Geometry: final body of the model. Coordinates: model frame, mm. Face numbers are marked on the shaded views. A direction names the side the tool comes from. Give positions to 0.01 mm unless a question says otherwise; leave off trailing zeros. Write each loop counter-clockwise with the first axis right and the second up, starting at its lowest first coordinate (ties: lowest second). Pieces come first, ordered by that corner, then holes. Notation, with made-up numbers: (22.5, 23.25) -> (29.5, 23.25) arc R18 ccw to (29.5, 35.25) -> close; hole circle Ø3 at (48, 72.25). An arc over 180 degrees is marked (long way). Answer as a JSON object with one key per item and string values.
from build123d import *

# Parameters (mm, degrees)
F1_DEPTH        = 10
F0_R            = 2.9
F2_DEPTH        = 3
F3_R            = 6.5
F4_DEPTH        = 4
F5_R            = 5
F6_DEPTH        = 12
F7_DEPTH        = 2
F8_D            = 3.3
F8_DEPTH        = 13.8
F8_START        = 2
F8_TIP          = 0.9914200214
F9_DEPTH        = 1.4
F10_D           = 3.3
F10_DEPTH       = 8
F10_TIP         = 0.9914200214
F12_D           = 3.3
F12_DEPTH       = 8
F12_CSINK_D     = 6.72
F12_CSINK_ANGLE = 90
F12_TIP         = 0.9914200214


with BuildPart() as f1:
    # F0 (on Front) → F1 (new body)
    with BuildSketch(Plane.XZ):
        with BuildLine():
            Line((20.9, 37.9), (17.9, 37.9))
            Line((17.9, 37.9), (-17.9, 37.9))
            Line((-17.9, 37.9), (-20.9, 37.9))
            ThreePointArc((-20.9, 37.9), (-22.3142135624, 37.3142135624), (-22.9, 35.9))
            Line((-22.9, 35.9), (-22.9, 32.9))
            Line((-22.9, 32.9), (-22.9, -35.9))
            ThreePointArc((-22.9, -35.9), (-22.3142135624, -37.3142135624), (-20.9, -37.9))
            Line((-20.9, -37.9), (20.9, -37.9))
            ThreePointArc((20.9, -37.9), (22.3142135624, -37.3142135624), (22.9, -35.9))
            Line((22.9, -35.9), (22.9, 32.9))
            Line((22.9, 32.9), (22.9, 35.9))
            ThreePointArc((22.9, 35.9), (22.3142135624, 37.3142135624), (20.9, 37.9))
        make_face()
        Polygon((7.4256842194, -31), (10.7743157806, -31), (12.4486315613, -33.9), (10.7743157806, -36.8), (7.4256842194, -36.8), (5.7513684387, -33.9), align=None, mode=Mode.SUBTRACT)
        Polygon((-16.2256842194, 36.8), (-14.5513684387, 33.9), (-16.2256842194, 31), (-19.5743157806, 31), (-21.2486315613, 33.9), (-19.5743157806, 36.8), align=None, mode=Mode.SUBTRACT)
        Polygon((20.9, 29.9), (20.9, -29.9), (18.3, -29.9), (-18.8811943151, -29.9), (-20.9, -29.9), (-20.9, 29.9), align=None, mode=Mode.SUBTRACT)
        Polygon((21.2486315613, 33.9), (19.5743157806, 31), (16.2256842194, 31), (14.5513684387, 33.9), (16.2256842194, 36.8), (19.5743157806, 36.8), align=None, mode=Mode.SUBTRACT)
        Polygon((-16.2256842194, 31), (-14.5513684387, 33.9), (-16.2256842194, 36.8), (-19.5743157806, 36.8), (-21.2486315613, 33.9), (-19.5743157806, 31), align=None)
        Polygon((16.2256842194, 31), (19.5743157806, 31), (21.2486315613, 33.9), (19.5743157806, 36.8), (16.2256842194, 36.8), (14.5513684387, 33.9), align=None)
        Polygon((12.4486315613, -33.9), (10.7743157806, -31), (7.4256842194, -31), (5.7513684387, -33.9), (7.4256842194, -36.8), (10.7743157806, -36.8), align=None)
    extrude(amount=F1_DEPTH)

    # F0 (on Front) → F2 (join)
    with BuildSketch(Plane.XZ):
        with BuildLine():
            Line((18.3, -29.9), (20.9, -29.9))
            Line((20.9, -29.9), (20.9, 29.9))
            Line((20.9, 29.9), (-20.9, 29.9))
            Line((-20.9, 29.9), (-20.9, -29.9))
            Line((-20.9, -29.9), (-18.8811943151, -29.9))
            Line((-18.8811943151, -29.9), (-18.8811943151, -20.7887917079))
            ThreePointArc((-18.8811943151, -20.7887917079), (-18.7640370276, -20.5059489954), (-18.4811943151, -20.3887917079))
            Line((-18.4811943151, -20.3887917079), (-17.9, -20.3887917079))
            ThreePointArc((-17.9, -20.3887917079), (-17.1928932188, -20.0958984891), (-16.9, -19.3887917079))
            Line((-16.9, -19.3887917079), (-16.9, -8))
            ThreePointArc((-16.9, -8), (-16.0213203436, -5.8786796564), (-13.9, -5))
            Line((-13.9, -5), (13.9, -5))
            ThreePointArc((13.9, -5), (16.0213203436, -5.8786796564), (16.9, -8))
            Line((16.9, -8), (16.9, -19.3887917079))
            ThreePointArc((16.9, -19.3887917079), (17.1928932188, -20.0958984891), (17.9, -20.3887917079))
            ThreePointArc((17.9, -20.3887917079), (18.1828427125, -20.5059489954), (18.3, -20.7887917079))
            Line((18.3, -20.7887917079), (18.3, -29.9))
        make_face()
        with Locations((-8.5, 0)):
            Circle(F0_R, mode=Mode.SUBTRACT)
        with Locations((8.5, 0)):
            Circle(F0_R, mode=Mode.SUBTRACT)
        with BuildLine():
            ThreePointArc((-16.9, 22.9), (-16.0213203436, 25.0213203436), (-13.9, 25.9))
            Line((-13.9, 25.9), (13.9, 25.9))
            ThreePointArc((13.9, 25.9), (16.0213203436, 25.0213203436), (16.9, 22.9))
            Line((16.9, 22.9), (16.9, 8))
            ThreePointArc((16.9, 8), (16.0213203436, 5.8786796564), (13.9, 5))
            Line((13.9, 5), (-13.9, 5))
            ThreePointArc((-13.9, 5), (-16.0213203436, 5.8786796564), (-16.9, 8))
            Line((-16.9, 8), (-16.9, 22.9))
        make_face(mode=Mode.SUBTRACT)
        with Locations((-8.5, 0)):
            Circle(F0_R)
        with Locations((8.5, 0)):
            Circle(F0_R)
    extrude(amount=F2_DEPTH)

    # F3 (on face) → F4 (cut)
    with BuildSketch(Plane.YZ.offset(22.9)):
        with Locations((-13.5, 17.9)):
            Circle(F3_R)
    extrude(amount=-F4_DEPTH, mode=Mode.SUBTRACT)

    # F5 (on face) → F6 (cut)
    with BuildSketch(Plane.XY.offset(37.9)):
        with Locations((-10.8651584014, -13)):
            Circle(F5_R)
    extrude(amount=-F6_DEPTH, mode=Mode.SUBTRACT)

    # F0 (on Front) → F7 (cut)
    with BuildSketch(Plane.XZ):
        Polygon((-16.2256842194, 31), (-14.5513684387, 33.9), (-16.2256842194, 36.8), (-19.5743157806, 36.8), (-21.2486315613, 33.9), (-19.5743157806, 31), align=None)
        Polygon((16.2256842194, 31), (19.5743157806, 31), (21.2486315613, 33.9), (19.5743157806, 36.8), (16.2256842194, 36.8), (14.5513684387, 33.9), align=None)
        Polygon((12.4486315613, -33.9), (10.7743157806, -31), (7.4256842194, -31), (5.7513684387, -33.9), (7.4256842194, -36.8), (10.7743157806, -36.8), align=None)
    extrude(amount=F7_DEPTH, mode=Mode.SUBTRACT)

    # F8
    # its depths count from where the whole tool has entered the part; down to there all is cleared
    with Locations(Plane(origin=(0, 0, 0), x_dir=(1, 0, 0), z_dir=(0, 1, 0)).offset(-F8_START)):
        with Locations((-17.9, -33.9), (17.9, -33.9), (9.1, 33.9)):
            Hole(F8_D / 2, depth=F8_DEPTH)
            with Locations((0, 0, -(F8_DEPTH + F8_TIP / 2))):  # 118° drill point
                Cone(0, F8_D / 2, F8_TIP, mode=Mode.SUBTRACT)

    # F0 (on Front) → F9 (join)
    with BuildSketch(Plane.XZ):
        with Locations((8.5, 0)):
            Circle(F0_R)
        with Locations((-8.5, 0)):
            Circle(F0_R)
    extrude(amount=-F9_DEPTH)

    # F10 (one way)
    with BuildSketch(Plane.XZ):
        with Locations((-8.5, 0), (8.5, 0)):
            Circle(F10_D / 2)
    extrude(amount=-F10_DEPTH, mode=Mode.SUBTRACT)
    with Locations(Plane.XZ):
        with Locations((-8.5, 0), (8.5, 0)):
            with Locations((0, 0, -(F10_DEPTH + F10_TIP / 2))):  # 118° drill point
                Cone(0, F10_D / 2, F10_TIP, mode=Mode.SUBTRACT)

    # F12
    with Locations(Plane.XZ.offset(3)):
        with Locations((-8.5, 0), (8.5, 0)):
            CounterSinkHole(F12_D / 2, F12_CSINK_D / 2, depth=F12_DEPTH, counter_sink_angle=F12_CSINK_ANGLE)
            with Locations((0, 0, -(F12_DEPTH + F12_TIP / 2))):  # 118° drill point
                Cone(0, F12_D / 2, F12_TIP, mode=Mode.SUBTRACT)


solid = f1.part
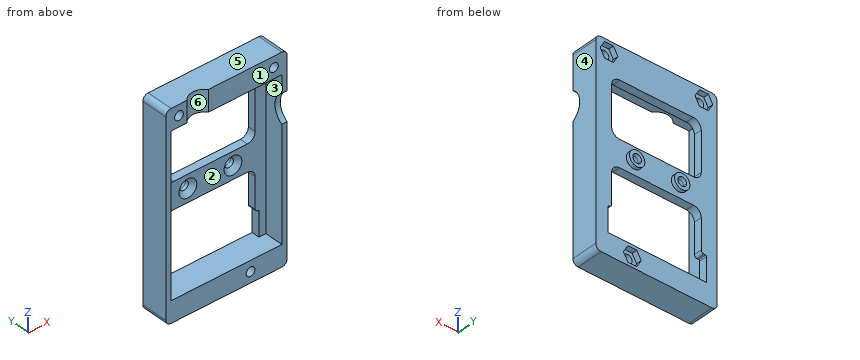
Q1. Cut plane C-C (y = -5.5). Return the cut outline in (x, z).
Values:
{"outline": "(-22.9, -35.9) arc R2 ccw to (-20.9, -37.9) -> (20.9, -37.9) arc R2 ccw to (22.9, -35.9) -> (22.9, 35.9) arc R2 ccw to (20.9, 37.9) -> (-20.9, 37.9) arc R2 ccw to (-22.9, 35.9) -> close; hole (-20.9, -29.9) -> (20.9, -29.9) -> (20.9, 29.9) -> (-20.9, 29.9) -> close; hole circle Ø3.3 at (-17.9, 33.9); hole circle Ø3.3 at (9.1, -33.9); hole circle Ø3.3 at (17.9, 33.9)"}
Q2. Material intervals for L1, parallel to Z at x = -8.5, y = -0.9; L2, parallel to X at y = -0.8, z = 0; L3, parallel to Z at x = 9.1, y = -5.5, sorted ascending. Write a range as from..to.
Values:
{"L1": "-37.9..-29.9, -5..-1.65, 1.65..5, 25.9..37.9", "L2": "-22.9..-10.15, -6.85..6.85, 10.15..22.9", "L3": "-37.9..-35.55, -32.25..-29.9, 29.9..37.9"}
Q3. Cut plane A-A (z = -14.5). Return the cut outline in (x, y), and give its area (3 significant figures).
Values:
{"outline": "(-22.9, -10) -> (-20.9, -10) -> (-20.9, -3) -> (-16.9, -3) -> (-16.9, 0) -> (-22.9, 0) -> close; (16.9, -3) -> (20.9, -3) -> (20.9, -10) -> (22.9, -10) -> (22.9, 0) -> (16.9, 0) -> close", "area": "64.0 mm²"}
Q4. Cut plane D-D (x = 8.5). State how many separate pieces and enclosed holes the cut face has, and give its area (3 significant figures).
Values:
{"separate pieces": "5", "enclosed holes": "0", "area": "156 mm²"}
Q5. First-contact query: P1, Ø3, axis at x = -17.5, z = 34.5, coming from the +Y side; P2, Ø4, axis at x = -6, z = -4, coming from the -Y side. Flat tips, straight axial feed; report the tip coordinate or a pass-through.
Values:
{"P1": "y = -2", "P2": "y = -3"}
Q6. Cut plane B-B (x = 2.5). Return the cut outline in (y, z), and give its area (3 significant figures).
Values:
{"outline": "(-10, -37.9) -> (0, -37.9) -> (0, -29.9) -> (-10, -29.9) -> close; (-10, 29.9) -> (-3, 29.9) -> (-3, 25.9) -> (0, 25.9) -> (0, 37.9) -> (-10, 37.9) -> close; (-3, -5) -> (0, -5) -> (0, 5) -> (-3, 5) -> close", "area": "202 mm²"}
Q7. Set-up query: the marked faces 5 and 6. Return all of +Z, -Z, +X, -X, +Y, -Y with unobstructed straight access to the full face (end or side cutting, diameter ignored); none if empty.
Values:
{"face 5": "+Z, +X, -X, +Y, -Y", "face 6": "+Z, -Y"}
Q8. Mould query, pull axis X, two halves, no side actions, for the marked faces 1, 2, 3 and 4. Classes: pulls with the +X half, pulls with the -X half, needs draft (parallel to the pull), parting line crosses it, or undercut.
Values:
{"face 1": "needs draft", "face 2": "undercut", "face 3": "undercut", "face 4": "pulls with the +X half"}
